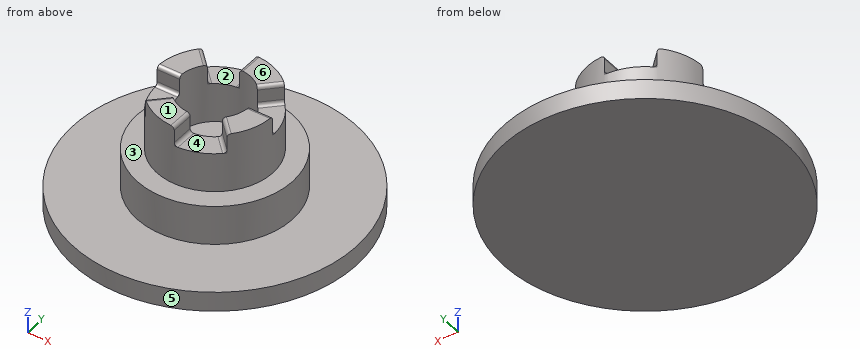
```python
from build123d import *

# Parameters (mm, degrees)
F0_R         = 10
F1_DEPTH     = 1.4
F2_R         = 5.5
F3_DEPTH     = 2.8
F4_R         = 4.1
F4_R_2       = 2.5
F5_DEPTH     = 4.2
F7_DEPTH     = 1.4
F8_T4_DEPTH  = 2.85
F8_S5_R      = 4.1
F8_T6_DEPTH  = 3
F8_S7_R      = 2.5
F8_T8_DEPTH  = 3
F8_T12_DEPTH = 2.85
F8_S13_R     = 4.1
F8_T14_DEPTH = 3
F8_S15_R     = 2.5
F8_T16_DEPTH = 3
F8_T20_DEPTH = 2.85
F8_S21_R     = 4.1
F8_T22_DEPTH = 3
F8_S23_R     = 2.5
F8_T24_DEPTH = 3
F8_T28_DEPTH = 2.85
F8_S29_R     = 4.1
F8_T30_DEPTH = 3
F8_S31_R     = 2.5
F8_T32_DEPTH = 3
F8_T36_DEPTH = 2.85
F8_S37_R     = 4.1
F8_T38_DEPTH = 3
F8_S39_R     = 2.5
F8_T40_DEPTH = 3
F8_T44_DEPTH = 2.85
F8_S45_R     = 4.1
F8_T46_DEPTH = 3
F8_S47_R     = 2.5
F8_T48_DEPTH = 3
F8_T52_DEPTH = 2.85
F8_S53_R     = 4.1
F8_T54_DEPTH = 3
F8_S55_R     = 2.5
F8_T56_DEPTH = 3
F8_T60_DEPTH = 2.85
F8_S61_R     = 4.1
F8_T62_DEPTH = 3
F8_S63_R     = 2.5
F8_T64_DEPTH = 3
F8_T65_DEPTH = 2.85
F8_T67_DEPTH = 2.85
F8_T69_DEPTH = 2.85
F8_T71_DEPTH = 2.85
F8_T73_DEPTH = 2.85
F8_T75_DEPTH = 2.85
F8_T77_DEPTH = 2.85
F8_T79_DEPTH = 2.85


# Not quite as in the source:
# - a fillet or chamfer that OpenCascade refuses, or shapes differently, is made with other operations: its cross-section is extruded or revolved along the edge and cut away or added


with BuildPart() as f1:
    # F0 (on Top) → F1 (new body)
    with BuildSketch(Plane.XY):
        Circle(F0_R)
    extrude(amount=F1_DEPTH)

    # F2 (on face) → F3 (join)
    with BuildSketch(Plane.XY.offset(1.4)):
        Circle(F2_R)
    extrude(amount=F3_DEPTH)

    # F4 (on face) → F5 (join)
    with BuildSketch(Plane.XY.offset(4.2)):
        Circle(F4_R)
        Circle(F4_R_2, mode=Mode.SUBTRACT)
    extrude(amount=F5_DEPTH)

    # F6 (on face) → F7 (cut)
    with BuildSketch(Plane.XY.offset(8.4)):
        with BuildLine():
            Line((0, -2.5), (0, -4.1))
            ThreePointArc((0, -4.1), (1.5690020727, -3.7879060833), (2.8991378029, -2.8991378029))
            Line((2.8991378029, -2.8991378029), (1.767766953, -1.767766953))
            ThreePointArc((1.767766953, -1.767766953), (0.9567085809, -2.3096988313), (0, -2.5))
        make_face()
        with BuildLine():
            ThreePointArc((-4.1, 0), (-3.7879060833, -1.5690020727), (-2.8991378029, -2.8991378029))
            Line((-2.8991378029, -2.8991378029), (-1.767766953, -1.767766953))
            ThreePointArc((-1.767766953, -1.767766953), (-2.3096988313, -0.9567085809), (-2.5, 0))
            Line((-2.5, 0), (-4.1, 0))
        make_face()
        with BuildLine():
            Line((2.5, 0), (4.1, 0))
            ThreePointArc((4.1, 0), (3.7879060833, 1.5690020727), (2.8991378029, 2.8991378029))
            Line((2.8991378029, 2.8991378029), (1.767766953, 1.767766953))
            ThreePointArc((1.767766953, 1.767766953), (2.3096988313, 0.9567085809), (2.5, 0))
        make_face()
        with BuildLine():
            ThreePointArc((-1.767766953, 1.767766953), (-0.9567085809, 2.3096988313), (0, 2.5))
            Line((0, 2.5), (0, 4.1))
            ThreePointArc((0, 4.1), (-1.5690020727, 3.7879060833), (-2.8991378029, 2.8991378029))
            Line((-2.8991378029, 2.8991378029), (-1.767766953, 1.767766953))
        make_face()
    extrude(amount=-F7_DEPTH, mode=Mode.SUBTRACT)

    # F8: fillet of radius 0.25 on 16 edges, made by hand


with BuildPart() as f8_tool2:
    # F8_s3 → F8_t4 (new body)
    with BuildSketch(Plane.YZ.offset(-1.875)):
        with BuildLine():
            ThreePointArc((-0.25, 7), (-0.0732233047, 7.0732233047), (0, 7.25))
            Line((0, 7.25), (0, 7))
            Line((0, 7), (-0.25, 7))
        make_face()
    extrude(amount=-F8_T4_DEPTH)

    # F8_s5 → F8_t6 (intersect, symmetric)
    with BuildSketch(Plane.XY.offset(7.1)):
        Circle(F8_S5_R)
    extrude(amount=F8_T6_DEPTH, both=True, mode=Mode.INTERSECT)

    # F8_s7 → F8_t8 (cut, symmetric)
    with BuildSketch(Plane.XY.offset(7.1)):
        Circle(F8_S7_R)
    extrude(amount=F8_T8_DEPTH, both=True, mode=Mode.SUBTRACT)


with BuildPart() as f1_1:
    add(f1.part)

    # F8_t1: union F8_tool2
    add(f8_tool2.part)


with BuildPart() as f8_tool10:
    # F8_s11 → F8_t12 (new body)
    with BuildSketch(Plane.XZ.offset(-1.875)):
        with BuildLine():
            ThreePointArc((-0.25, 7), (-0.0732233047, 7.0732233047), (0, 7.25))
            Line((0, 7.25), (0, 7))
            Line((0, 7), (-0.25, 7))
        make_face()
    extrude(amount=-F8_T12_DEPTH)

    # F8_s13 → F8_t14 (intersect, symmetric)
    with BuildSketch(Plane.XY.offset(7.1)):
        Circle(F8_S13_R)
    extrude(amount=F8_T14_DEPTH, both=True, mode=Mode.INTERSECT)

    # F8_s15 → F8_t16 (cut, symmetric)
    with BuildSketch(Plane.XY.offset(7.1)):
        Circle(F8_S15_R)
    extrude(amount=F8_T16_DEPTH, both=True, mode=Mode.SUBTRACT)


with BuildPart() as f1_2:
    add(f1_1.part)

    # F8_t9: union F8_tool10
    add(f8_tool10.part)


with BuildPart() as f8_tool18:
    # F8_s19 → F8_t20 (new body)
    with BuildSketch(Plane(origin=(3.3410795411, -3.3410795411, 0), x_dir=(0, 0, 1), z_dir=(-0.7071067812, 0.7071067812, 0))):
        with BuildLine():
            ThreePointArc((7.25, 0), (7.0732233047, -0.0732233047), (7, -0.25))
            Line((7, -0.25), (7, 0))
            Line((7, 0), (7.25, 0))
        make_face()
    extrude(amount=F8_T20_DEPTH)

    # F8_s21 → F8_t22 (intersect, symmetric)
    with BuildSketch(Plane.XY.offset(7.1)):
        Circle(F8_S21_R)
    extrude(amount=F8_T22_DEPTH, both=True, mode=Mode.INTERSECT)

    # F8_s23 → F8_t24 (cut, symmetric)
    with BuildSketch(Plane.XY.offset(7.1)):
        Circle(F8_S23_R)
    extrude(amount=F8_T24_DEPTH, both=True, mode=Mode.SUBTRACT)


with BuildPart() as f1_3:
    add(f1_2.part)

    # F8_t17: union F8_tool18
    add(f8_tool18.part)


with BuildPart() as f8_tool26:
    # F8_s27 → F8_t28 (new body)
    with BuildSketch(Plane.YZ.offset(1.875)):
        with BuildLine():
            ThreePointArc((0, 7.25), (0.0732233047, 7.0732233047), (0.25, 7))
            Line((0.25, 7), (0, 7))
            Line((0, 7), (0, 7.25))
        make_face()
    extrude(amount=F8_T28_DEPTH)

    # F8_s29 → F8_t30 (intersect, symmetric)
    with BuildSketch(Plane.XY.offset(7.1)):
        Circle(F8_S29_R)
    extrude(amount=F8_T30_DEPTH, both=True, mode=Mode.INTERSECT)

    # F8_s31 → F8_t32 (cut, symmetric)
    with BuildSketch(Plane.XY.offset(7.1)):
        Circle(F8_S31_R)
    extrude(amount=F8_T32_DEPTH, both=True, mode=Mode.SUBTRACT)


with BuildPart() as f1_4:
    add(f1_3.part)

    # F8_t25: union F8_tool26
    add(f8_tool26.part)


with BuildPart() as f8_tool34:
    # F8_s35 → F8_t36 (new body)
    with BuildSketch(Plane(origin=(-3.3410795411, -3.3410795411, 0), x_dir=(0, 0, 1), z_dir=(0.7071067812, 0.7071067812, 0))):
        with BuildLine():
            ThreePointArc((7.25, 0), (7.0732233047, -0.0732233047), (7, -0.25))
            Line((7, -0.25), (7, 0))
            Line((7, 0), (7.25, 0))
        make_face()
    extrude(amount=F8_T36_DEPTH)

    # F8_s37 → F8_t38 (intersect, symmetric)
    with BuildSketch(Plane.XY.offset(7.1)):
        Circle(F8_S37_R)
    extrude(amount=F8_T38_DEPTH, both=True, mode=Mode.INTERSECT)

    # F8_s39 → F8_t40 (cut, symmetric)
    with BuildSketch(Plane.XY.offset(7.1)):
        Circle(F8_S39_R)
    extrude(amount=F8_T40_DEPTH, both=True, mode=Mode.SUBTRACT)


with BuildPart() as f1_5:
    add(f1_4.part)

    # F8_t33: union F8_tool34
    add(f8_tool34.part)


with BuildPart() as f8_tool42:
    # F8_s43 → F8_t44 (new body)
    with BuildSketch(Plane(origin=(-3.3410795411, 3.3410795411, 0), x_dir=(0, 0, 1), z_dir=(0.7071067812, -0.7071067812, 0))):
        with BuildLine():
            ThreePointArc((7.25, 0), (7.0732233047, -0.0732233047), (7, -0.25))
            Line((7, -0.25), (7, 0))
            Line((7, 0), (7.25, 0))
        make_face()
    extrude(amount=F8_T44_DEPTH)

    # F8_s45 → F8_t46 (intersect, symmetric)
    with BuildSketch(Plane.XY.offset(7.1)):
        Circle(F8_S45_R)
    extrude(amount=F8_T46_DEPTH, both=True, mode=Mode.INTERSECT)

    # F8_s47 → F8_t48 (cut, symmetric)
    with BuildSketch(Plane.XY.offset(7.1)):
        Circle(F8_S47_R)
    extrude(amount=F8_T48_DEPTH, both=True, mode=Mode.SUBTRACT)


with BuildPart() as f1_6:
    add(f1_5.part)

    # F8_t41: union F8_tool42
    add(f8_tool42.part)


with BuildPart() as f8_tool50:
    # F8_s51 → F8_t52 (new body)
    with BuildSketch(Plane.XZ.offset(1.875)):
        with BuildLine():
            ThreePointArc((0.25, 7), (0.0732233047, 7.0732233047), (0, 7.25))
            Line((0, 7.25), (0, 7))
            Line((0, 7), (0.25, 7))
        make_face()
    extrude(amount=F8_T52_DEPTH)

    # F8_s53 → F8_t54 (intersect, symmetric)
    with BuildSketch(Plane.XY.offset(7.1)):
        Circle(F8_S53_R)
    extrude(amount=F8_T54_DEPTH, both=True, mode=Mode.INTERSECT)

    # F8_s55 → F8_t56 (cut, symmetric)
    with BuildSketch(Plane.XY.offset(7.1)):
        Circle(F8_S55_R)
    extrude(amount=F8_T56_DEPTH, both=True, mode=Mode.SUBTRACT)


with BuildPart() as f1_7:
    add(f1_6.part)

    # F8_t49: union F8_tool50
    add(f8_tool50.part)


with BuildPart() as f8_tool58:
    # F8_s59 → F8_t60 (new body)
    with BuildSketch(Plane(origin=(3.3410795411, 3.3410795411, 0), x_dir=(0, 0, 1), z_dir=(-0.7071067812, -0.7071067812, 0))):
        with BuildLine():
            ThreePointArc((7.25, 0), (7.0732233047, -0.0732233047), (7, -0.25))
            Line((7, -0.25), (7, 0))
            Line((7, 0), (7.25, 0))
        make_face()
    extrude(amount=F8_T60_DEPTH)

    # F8_s61 → F8_t62 (intersect, symmetric)
    with BuildSketch(Plane.XY.offset(7.1)):
        Circle(F8_S61_R)
    extrude(amount=F8_T62_DEPTH, both=True, mode=Mode.INTERSECT)

    # F8_s63 → F8_t64 (cut, symmetric)
    with BuildSketch(Plane.XY.offset(7.1)):
        Circle(F8_S63_R)
    extrude(amount=F8_T64_DEPTH, both=True, mode=Mode.SUBTRACT)


with BuildPart() as f1_8:
    add(f1_7.part)

    # F8_t57: union F8_tool58
    add(f8_tool58.part)

    # F8_s66 → F8_t65 (cut)
    with BuildSketch(Plane.YZ.offset(-4.725)):
        with BuildLine():
            ThreePointArc((0, 8.15), (0.0732233047, 8.3267766953), (0.25, 8.4))
            Line((0.25, 8.4), (0, 8.4))
            Line((0, 8.4), (0, 8.15))
        make_face()
    extrude(amount=F8_T65_DEPTH, mode=Mode.SUBTRACT)

    # F8_s68 → F8_t67 (cut)
    with BuildSketch(Plane(origin=(-3.3410795411, 3.3410795411, 0), x_dir=(0, 0, 1), z_dir=(0.7071067812, -0.7071067812, 0))):
        with BuildLine():
            ThreePointArc((8.4, 0.25), (8.3267766953, 0.0732233047), (8.15, 0))
            Line((8.15, 0), (8.4, 0))
            Line((8.4, 0), (8.4, 0.25))
        make_face()
    extrude(amount=F8_T67_DEPTH, mode=Mode.SUBTRACT)

    # F8_s70 → F8_t69 (cut)
    with BuildSketch(Plane.XZ.offset(1.875)):
        with BuildLine():
            ThreePointArc((0, 8.15), (-0.0732233047, 8.3267766953), (-0.25, 8.4))
            Line((-0.25, 8.4), (0, 8.4))
            Line((0, 8.4), (0, 8.15))
        make_face()
    extrude(amount=F8_T69_DEPTH, mode=Mode.SUBTRACT)

    # F8_s72 → F8_t71 (cut)
    with BuildSketch(Plane(origin=(-3.3410795411, -3.3410795411, 0), x_dir=(0, 0, 1), z_dir=(0.7071067812, 0.7071067812, 0))):
        with BuildLine():
            ThreePointArc((8.4, 0.25), (8.3267766953, 0.0732233047), (8.15, 0))
            Line((8.15, 0), (8.4, 0))
            Line((8.4, 0), (8.4, 0.25))
        make_face()
    extrude(amount=F8_T71_DEPTH, mode=Mode.SUBTRACT)

    # F8_s74 → F8_t73 (cut)
    with BuildSketch(Plane.YZ.offset(1.875)):
        with BuildLine():
            ThreePointArc((0, 8.15), (-0.0732233047, 8.3267766953), (-0.25, 8.4))
            Line((-0.25, 8.4), (0, 8.4))
            Line((0, 8.4), (0, 8.15))
        make_face()
    extrude(amount=F8_T73_DEPTH, mode=Mode.SUBTRACT)

    # F8_s76 → F8_t75 (cut)
    with BuildSketch(Plane(origin=(3.3410795411, -3.3410795411, 0), x_dir=(0, 0, 1), z_dir=(-0.7071067812, 0.7071067812, 0))):
        with BuildLine():
            ThreePointArc((8.4, 0.25), (8.3267766953, 0.0732233047), (8.15, 0))
            Line((8.15, 0), (8.4, 0))
            Line((8.4, 0), (8.4, 0.25))
        make_face()
    extrude(amount=F8_T75_DEPTH, mode=Mode.SUBTRACT)

    # F8_s78 → F8_t77 (cut)
    with BuildSketch(Plane.XZ.offset(-4.725)):
        with BuildLine():
            ThreePointArc((0, 8.15), (0.0732233047, 8.3267766953), (0.25, 8.4))
            Line((0.25, 8.4), (0, 8.4))
            Line((0, 8.4), (0, 8.15))
        make_face()
    extrude(amount=F8_T77_DEPTH, mode=Mode.SUBTRACT)

    # F8_s80 → F8_t79 (cut)
    with BuildSketch(Plane(origin=(3.3410795411, 3.3410795411, 0), x_dir=(0, 0, 1), z_dir=(-0.7071067812, -0.7071067812, 0))):
        with BuildLine():
            ThreePointArc((8.4, 0.25), (8.3267766953, 0.0732233047), (8.15, 0))
            Line((8.15, 0), (8.4, 0))
            Line((8.4, 0), (8.4, 0.25))
        make_face()
    extrude(amount=F8_T79_DEPTH, mode=Mode.SUBTRACT)


solid = f1_8.part
```
Source: CAD feature listing. Evaluate the final solid. Frame: model axes, mm. Face numbers are marked on the shaded views. A direction names the side the tool comes from. Coordinates: 2 decimals unless noted, no trailing zeros. Loops run counter-clockwise (first coordinate to the right, second up) from the corner with the lowest first, then second, coordinate; pieces in that order, holes last. Notation, with made-up numbers: M 23.25,-21 L 38.25,-21 A19 ccw 38.25,1 Z; hole C -35,-8.5 d1. An arc over 180 degrees is marked long. Put each result on its own line as item: value. Start each with the question number.
1) Cut plane D-D on z = 1. Return the cut outline in (x, y).
2) Cut plane B-B on y = 3.75. Return the cut outline in (x, z), then the cut area to 3 significant figures.
3) Ray query, L1, parallel to Y at x = 0, z = 5.1; L2, parallel to Z at x = -3, y = 8.5; L3, parallel to Z at x = 1, y = -2. Return the intervals inside material, ascending. Write a range as from..to.
4) Pull-direction query (X, two-part tool) for the marked faces 4, 5 and 6; classes: pulls with the +X half, pulls with the -X half, needs draft (parallel to the pull), parting line crosses it, or undercut.
5) Cut plane C-C on x = 1.25. Return the cut outline in (y, z), then the cut area to 3 significant figures.
6) Cut plane A-A on z = 4.5. Return the cut outline in (x, y), then the cut area to 3 significant figures.
7) Reachability of the marked faces 1, 2 and 3 from +Z, -Z, +X, -X, +Y, -Y: full face, straight path, thin tool, end or side. Return the list, or none.
8) Contact query for flat-ended pins moving along their axis: pin 1 Ø1 at (x, z) = (-1, 4.5) entering from -Y; pin 2 Ø0.6 at (x, y) = (-3, -1.5) entering from +Z; pin 3 Ø1.5 at (x, z) = (-2, 6) entering from +Y. Output: stop coordinate, or through.
The answers:
1. outline: C 0,0 d20
2. outline: M -9.27,0 L 9.27,0 L 9.27,1.4 L 4.02,1.4 L 4.02,4.2 L 1.66,4.2 L 1.66,8.4 L 0.25,8.4 A0.25 ccw 0,8.15 L 0,7.25 A0.25 cw -0.25,7 L -1.66,7 L -1.66,4.2 L -4.02,4.2 L -4.02,1.4 L -9.27,1.4 Z
2. area: 60.1 mm²
3. L1: y = -4.1..-2.5, 2.5..4.1
3. L2: z = 0..1.4
3. L3: z = 0..4.2
4. face 4: undercut
4. face 5: parting line crosses it
4. face 6: needs draft
5. outline: M -9.92,0 L 9.92,0 L 9.92,1.4 L 5.36,1.4 L 5.36,4.2 L 3.9,4.2 L 3.9,8.4 L 2.17,8.4 L 2.17,4.2 L -2.17,4.2 L -2.17,7 L -3.9,7 L -3.9,4.2 L -5.36,4.2 L -5.36,1.4 L -9.92,1.4 Z
5. area: 70.0 mm²
6. outline: C 0,0 d8.2; hole C 0,0 d5
6. area: 33.2 mm²
7. face 1: +Z, +X, -X, +Y, -Y
7. face 2: +Z, +Y
7. face 3: +Z
8. pin 1: stops at y = -5.47
8. pin 2: stops at z = 7
8. pin 3: stops at y = 3.9
